CAD build for the part. Positions are in the model's coordinates, mm. A direction names the side the tool comes from. Coordinates: 2 decimals unless noted, no trailing zeros. Write each loop counter-clockwise with the first axis right and the second up, starting at its lowest first coordinate (ties: lowest second). Pieces come first, ordered by that corner, then holes. Notation, with made-up numbers: (23, 65.25) -> (41, 65.25) arc R30 cw to (41, 93.25) -> close; hole circle Ø6 at (77, 21). An arc over 180 degrees is marked (long way). Answer as CSV lines item,"result". Start each with the question number.
```python
from build123d import *

# Parameters (mm, degrees)
SKETCH1_W           = 6
SKETCH1_H           = 6
BOSS_EXTRUDE1_DEPTH = 6
SKETCH2_W           = 12
SKETCH2_H           = 6
BOSS_EXTRUDE2_DEPTH = 3
SKETCH3_W           = 2
SKETCH3_H           = 6
BOSS_EXTRUDE3_DEPTH = 2.5


with BuildPart() as part:
    # Sketch1 → Boss-Extrude1 (new body)
    with BuildSketch(Plane(origin=(0, 0, 0), x_dir=(1, 0, 0), z_dir=(0, 1, 0))):
        Rectangle(SKETCH1_W, SKETCH1_H)
    extrude(amount=BOSS_EXTRUDE1_DEPTH)

    # Sketch2 → Boss-Extrude2 (add)
    with BuildSketch(Plane(origin=(0, 6, 0), x_dir=(1, 0, 0), z_dir=(0, 1, 0))):
        with Locations((-3, 0)):
            Rectangle(SKETCH2_W, SKETCH2_H)
    extrude(amount=BOSS_EXTRUDE2_DEPTH)

    # Sketch3 → Boss-Extrude3 (add)
    with BuildSketch(Plane.XZ.offset(-6)):
        with Locations((-8, 0)):
            Rectangle(SKETCH3_W, SKETCH3_H)
    extrude(amount=BOSS_EXTRUDE3_DEPTH)


solid = part.part
```
1. Tool access for faces 1 (the face through (-7, 5, 0)), 2 (the face through (-8, 3.5, 0)), 3 (the face through (-9, 6, 0)): list every direction of +Z, -Z, +X, -X, +Y, -Y with a clear straight run to the whole face (end or side of a thin tool).
2. Cut at B-B (z = -0.2). Give the cut face in (x, y), then the cut area to 3 significant figures.
3. Mould opens along X. For faces 4 (the face through (3, 4, 0)), 5 (the face through (-5, 6, 0)), 6 (the face through (-2, 6, 3)) say: pulls with the +X half, pulls with the -X half, needs draft (parallel to the pull), parting line crosses it, or undercut.
4. Wall check: line 1 (X direction, y = 2.25, z = -0.05); line 2 (Y direction, x = -6, z = -0.6). Give the ranges that are in metal, low to high.
5. Cut at A-A (y = 4.25). Give the cut face in (x, z).
6. Cut at C-C (y = 3). Give the cut face in (x, z).
7. Flat gauge pin, fed straight in: P1, Ø2, axis at x = -8.5, z = -1, coming from the -Y side. Where does the tip first touch, or does it go through?
8. Cut at D-D (x = -6.25). Give the cut face in (y, z).
Geometry check:
1,face 1,"+Z, -Z, -Y"
1,face 2,"+Z, -Z, -X, -Y"
1,face 3,"+Z, -Z, -X, +Y, -Y"
2,outline,"(-9, 3.5) -> (-7, 3.5) -> (-7, 6) -> (-3, 6) -> (-3, 0) -> (3, 0) -> (3, 9) -> (-9, 9) -> close"
2,area,"77.0 mm²"
3,face 4,"pulls with the +X half"
3,face 5,"undercut"
3,face 6,"needs draft"
4,line 1,"-3 to 3"
4,line 2,"6 to 9"
5,outline,"(-9, -3) -> (-7, -3) -> (-7, 3) -> (-9, 3) -> close; (-3, -3) -> (3, -3) -> (3, 3) -> (-3, 3) -> close"
6,outline,"(-3, -3) -> (3, -3) -> (3, 3) -> (-3, 3) -> close"
7,P1,"y = 3.5"
8,outline,"(6, -3) -> (9, -3) -> (9, 3) -> (6, 3) -> close"
